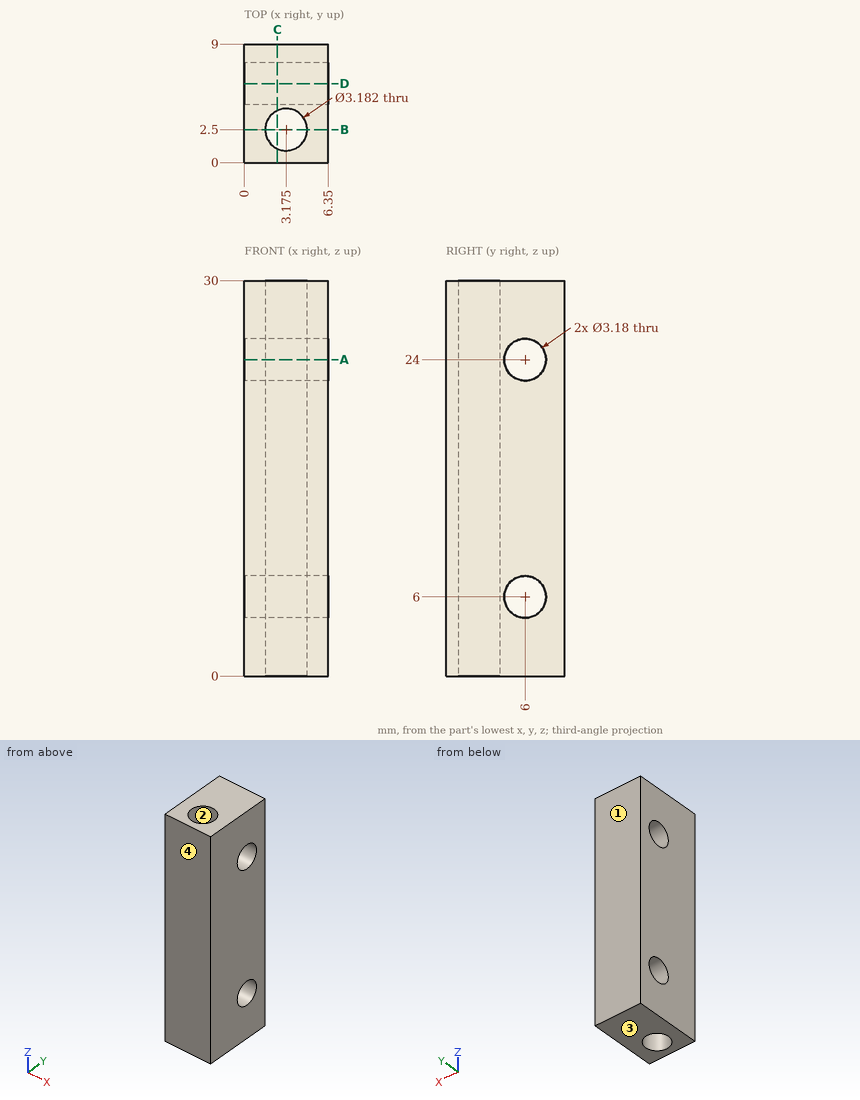
The drawing under review shows one solid part. Ordinate dimensions are in mm from its lowest x, y, z. Coordinates: 2 decimals unless noted, no trailing zeros. Write each loop counter-clockwise with the first axis right and the second up, starting at its lowest first coordinate (ties: lowest second). Pieces come first, ordered by that corner, then holes. Notation, with made-up numbers: (48, 30) - (102, 30) arc R24 ccw to (102, 59) - close; hole circle Ø7 at (16.25, -7). An arc over 180 degrees is marked (long way). Use one line per item in the form item = value.
Q1. Consider section D-D (y = 6). Write out the cut boundary in (x, z).
Taken from the geometry:
outline = (0, 0) - (6.35, 0) - (6.35, 4.41) - (0, 4.41) - close; (0, 7.59) - (6.35, 7.59) - (6.35, 22.41) - (0, 22.41) - close; (0, 25.59) - (6.35, 25.59) - (6.35, 30) - (0, 30) - close
Q2. Consider section C-C (x = 2.5). Write out the cut boundary in (y, z).
Taken from the geometry:
outline = (0, 0) - (1.06, 0) - (1.06, 30) - (0, 30) - close; (3.94, 0) - (9, 0) - (9, 30) - (3.94, 30) - close; hole circle Ø3.18 at (6, 6); hole circle Ø3.18 at (6, 24)
Q3. The part is to be moulded in two halves that separate along Y. For the marked faces 1, 2, 3 and 4, say which applies: +Y half, -Y half, draft (parallel to the pull), parting line (faces both ways), or undercut.
Taken from the geometry:
face_1 = +Y half
face_2 = undercut
face_3 = draft
face_4 = -Y half
Q4. Consider section A-A (z = 24). Write out the cut boundary in (x, y) (3 decimals), plus the area to 3 significant figures.
Taken from the geometry:
outline = (0, 0) - (6.35, 0) - (6.35, 4.41) - (0, 4.41) - close; (0, 7.59) - (6.35, 7.59) - (6.35, 9) - (0, 9) - close; hole circle Ø3.182 at (3.175, 2.5)
area = 29.0 mm^2
Q5. For probe 1 along Z at (x, y) = (4.25, 6); probe 2 along Z at (x, y) = (3.5, 5); probe 3 along Y at (x, z) = (4, 24), list the stretches that pass through material, from the lowest coordinate up.
Taken from the geometry:
probe_1 = 0 to 4.41, 7.59 to 22.41, 25.59 to 30
probe_2 = 0 to 4.76, 7.24 to 22.76, 25.24 to 30
probe_3 = 0 to 1.14, 3.86 to 4.41, 7.59 to 9
Q6. Consider section B-B (y = 2.5). Write out the cut boundary in (x, z).
Taken from the geometry:
outline = (0, 0) - (1.58, 0) - (1.58, 30) - (0, 30) - close; (4.77, 0) - (6.35, 0) - (6.35, 30) - (4.77, 30) - close
